Check sheet for the modelled part. Datum: model origin and axes. Units: mm. Round coordinates to 2 decimals unless told otherwise and drop trailing zeros. Write each loop counter-clockwise with the first axis right and the second up, starting at its lowest first coordinate (ties: lowest second). Pieces come first, ordered by that corner, then holes.
Item 1: Cross-section at B-B on y = 104.65. Count the separate pieces of the cut face and the enclosed holes in it, plus the area to 3 significant figures.
Item 2: Go/stop test with flat-tipped pins: pin 1 Ø1.2 at (x, y) = (109, 103) entering from -Z; pin 2 Ø1.2 at (x, y) = (141, 103.5) entering from -Z; pin 3 Ø1 at (y, z) = (104, 218) entering from -X. Record where each tip stops, or that it passes through.
Item 3: Material ranges on line 1 (Z direction, x = 67, y = 103.9); line 2 (Z direction, x = 188.5, y = 103.75); line 3 (Z direction, x = 170.5, y = 101.6), recorded low to high.
Item 4: Cross-section at A-A on x = 77.5. Enter the section's corners in (y, z), plus the area to 3 significant figures.
Item 5: Cross-section at C-C on x = 134. Enter the section's corners in (y, z).
from build123d import *

# Parameters (mm, degrees)
SKETCH1_W           = 10.75
SKETCH1_H           = 4
SKETCH1_R           = 1.6
SKETCH1_R_2         = 9
SKETCH1_R_3         = 8.5
BOSS_EXTRUDE1_DEPTH = 4
FILLET2_R           = 3


with BuildPart() as part:
    # Sketch1 → Boss-Extrude1 (new body)
    with BuildSketch(Plane(origin=(0, 101.33365526, 0), x_dir=(1, 0, 0), z_dir=(0, 1, 0))):
        with BuildLine():
            Line((99.937186027, -237.061198021), (99.937186027, -207.061198021))
            Line((99.937186027, -207.061198021), (112.937186027, -207.061198021))
            Line((112.937186027, -207.061198021), (112.937186027, -193.701198021))
            Line((112.937186027, -193.701198021), (116.937186027, -193.701198021))
            Line((116.937186027, -193.701198021), (116.937186027, -193.724971735))
            ThreePointArc((116.937186027, -193.724971735), (120.422613168, -188.743411519), (125.937186027, -186.183405518))
            Line((125.937186027, -186.183405518), (125.937186027, -182.011198021))
            Line((125.937186027, -182.011198021), (129.937186027, -182.011198021))
            Line((129.937186027, -182.011198021), (129.937186027, -186.183405518))
            ThreePointArc((129.937186027, -186.183405518), (135.451758886, -188.743411519), (138.937186027, -193.724971735))
            Line((138.937186027, -193.724971735), (138.937186027, -193.701198021))
            Line((138.937186027, -193.701198021), (142.937186027, -193.701198021))
            Line((142.937186027, -193.701198021), (142.937186027, -207.061198021))
            Line((142.937186027, -207.061198021), (155.937186027, -207.061198021))
            Line((155.937186027, -207.061198021), (155.937186027, -237.061198021))
            Line((155.937186027, -237.061198021), (180.437186027, -237.061198021))
            ThreePointArc((180.437186027, -237.061198021), (216.632797463, -160.061198021), (180.437186027, -83.061198021))
            Line((180.437186027, -83.061198021), (155.937186027, -83.061198021))
            Line((155.937186027, -83.061198021), (155.937186027, -113.061198021))
            Line((155.937186027, -113.061198021), (142.937186027, -113.061198021))
            Line((142.937186027, -113.061198021), (142.937186027, -126.421198021))
            Line((142.937186027, -126.421198021), (138.937186027, -126.421198021))
            Line((138.937186027, -126.421198021), (138.937186027, -126.397424307))
            ThreePointArc((138.937186027, -126.397424307), (135.451758886, -131.378984523), (129.937186027, -133.938990524))
            Line((129.937186027, -133.938990524), (129.937186027, -138.111198021))
            Line((129.937186027, -138.111198021), (125.937186027, -138.111198021))
            Line((125.937186027, -138.111198021), (125.937186027, -133.938990524))
            ThreePointArc((125.937186027, -133.938990524), (120.422613168, -131.378984523), (116.937186027, -126.397424307))
            Line((116.937186027, -126.397424307), (116.937186027, -126.421198021))
            Line((116.937186027, -126.421198021), (112.937186027, -126.421198021))
            Line((112.937186027, -126.421198021), (112.937186027, -113.061198021))
            Line((112.937186027, -113.061198021), (99.937186027, -113.061198021))
            Line((99.937186027, -113.061198021), (99.937186027, -83.061198021))
            Line((99.937186027, -83.061198021), (52.828408899, -83.061198021))
            ThreePointArc((52.828408899, -83.061198021), (16.632797463, -160.061198021), (52.828408899, -237.061198021))
            Line((52.828408899, -237.061198021), (99.937186027, -237.061198021))
        make_face()
        with Locations((175.062186027, -95.061198021)):
            Rectangle(SKETCH1_W, SKETCH1_H, mode=Mode.SUBTRACT)
        Polygon((56.893376849, -220.531213103), (49.699978846, -227.477796808), (46.921345364, -224.600437606), (54.114743367, -217.653853902), align=None, mode=Mode.SUBTRACT)
        with Locations((104.217909851, -196.061198021)):
            Circle(SKETCH1_R, mode=Mode.SUBTRACT)
        Polygon((116.937186027, -142.561198021), (116.937186027, -177.561198021), (112.937186027, -177.561198021), (112.937186027, -162.061198021), (106.437186027, -162.061198021), (106.437186027, -158.061198021), (112.937186027, -158.061198021), (112.937186027, -142.561198021), align=None, mode=Mode.SUBTRACT)
        with Locations((175.062186027, -225.061198021)):
            Rectangle(SKETCH1_W, SKETCH1_H, mode=Mode.SUBTRACT)
        with Locations((175.937186027, -203.061198021)):
            Circle(SKETCH1_R_2, mode=Mode.SUBTRACT)
        Polygon((192.781361608, -217.850313996), (189.504753431, -215.55600825), (191.799059176, -212.279400073), (195.075667353, -214.573705818), align=None, mode=Mode.SUBTRACT)
        Polygon((201.615472458, -203.246431106), (197.990241309, -201.555958059), (199.680714356, -197.930726911), (203.305945504, -199.621199958), align=None, mode=Mode.SUBTRACT)
        with Locations((162.937186027, -190.561198021)):
            Circle(SKETCH1_R, mode=Mode.SUBTRACT)
        Polygon((138.937186027, -142.561198021), (142.937186027, -142.561198021), (142.937186027, -158.061198021), (149.437186027, -158.061198021), (149.437186027, -162.061198021), (142.937186027, -162.061198021), (142.937186027, -177.561198021), (138.937186027, -177.561198021), align=None, mode=Mode.SUBTRACT)
        with Locations((188.937186027, -190.561198021)):
            Circle(SKETCH1_R, mode=Mode.SUBTRACT)
        Polygon((173.937186027, -138.161198021), (173.937186027, -134.961198021), (177.937186027, -134.961198021), (177.937186027, -138.161198021), (187.387186027, -138.161198021), (187.387186027, -158.061198021), (188.887186027, -158.061198021), (188.887186027, -162.061198021), (187.387186027, -162.061198021), (187.387186027, -181.961198021), (177.937186027, -181.961198021), (177.937186027, -185.161198021), (173.937186027, -185.161198021), (173.937186027, -181.961198021), (164.487186027, -181.961198021), (164.487186027, -138.161198021), align=None, mode=Mode.SUBTRACT)
        Polygon((211.08596232, -170.585781918), (207.101183528, -170.237158947), (207.449806499, -166.252380154), (211.434585291, -166.601003125), align=None, mode=Mode.SUBTRACT)
        with BuildLine():
            ThreePointArc((30.129612814, -122.561198021), (32.472758565, -116.904343772), (38.129612814, -114.561198021))
            Line((38.129612814, -114.561198021), (46.129612814, -114.561198021))
            ThreePointArc((46.129612814, -114.561198021), (51.786467064, -116.904343772), (54.129612814, -122.561198021))
            Line((54.129612814, -122.561198021), (54.129612814, -197.561198021))
            ThreePointArc((54.129612814, -197.561198021), (51.786467064, -203.21805227), (46.129612814, -205.561198021))
            Line((46.129612814, -205.561198021), (38.129612814, -205.561198021))
            ThreePointArc((38.129612814, -205.561198021), (32.472758565, -203.21805227), (30.129612814, -197.561198021))
            Line((30.129612814, -197.561198021), (30.129612814, -122.561198021))
        make_face(mode=Mode.SUBTRACT)
        with BuildLine():
            Line((58.629612814, -206.061198021), (58.629612814, -114.061198021))
            Line((58.629612814, -114.061198021), (80.629612814, -114.061198021))
            ThreePointArc((80.629612814, -114.061198021), (82.750933158, -114.939877677), (83.629612814, -117.061198021))
            Line((83.629612814, -117.061198021), (83.629612814, -203.061198021))
            ThreePointArc((83.629612814, -203.061198021), (82.750933158, -205.182518365), (80.629612814, -206.061198021))
            Line((80.629612814, -206.061198021), (58.629612814, -206.061198021))
        make_face(mode=Mode.SUBTRACT)
        with Locations((104.217909851, -124.061198021)):
            Circle(SKETCH1_R, mode=Mode.SUBTRACT)
        Polygon((54.114743367, -102.46854214), (46.921345364, -95.521958436), (49.699978846, -92.644599234), (56.893376849, -99.591182939), align=None, mode=Mode.SUBTRACT)
        with Locations((127.937186027, -160.061198021)):
            Circle(SKETCH1_R_3, mode=Mode.SUBTRACT)
        with Locations((162.937186027, -129.561198021)):
            Circle(SKETCH1_R, mode=Mode.SUBTRACT)
        Polygon((211.434585291, -153.521392917), (207.449806499, -153.870015888), (207.101183528, -149.885237095), (211.08596232, -149.536614124), align=None, mode=Mode.SUBTRACT)
        with Locations((188.937186027, -129.561198021)):
            Circle(SKETCH1_R, mode=Mode.SUBTRACT)
        with Locations((175.937186027, -117.061198021)):
            Circle(SKETCH1_R_2, mode=Mode.SUBTRACT)
        Polygon((203.305945504, -120.501196084), (199.680714356, -122.191669131), (197.990241309, -118.566437983), (201.615472457, -116.875964936), align=None, mode=Mode.SUBTRACT)
        Polygon((195.075667353, -105.548690224), (191.799059176, -107.842995969), (189.504753431, -104.566387792), (192.781361608, -102.272082046), align=None, mode=Mode.SUBTRACT)
    extrude(amount=BOSS_EXTRUDE1_DEPTH)

    # Fillet2
    fillet2_edges = [part.edges().sort_by_distance(p)[0] for p in [
        (99.937186027, 103.33365526, 83.061198021),
        (99.937186027, 103.33365526, 113.061198021),
        (155.937186027, 103.33365526, 113.061198021),
        (155.937186027, 103.33365526, 83.061198021),
        (155.937186027, 103.33365526, 237.061198021),
        (155.937186027, 103.33365526, 207.061198021),
        (99.937186027, 103.33365526, 207.061198021),
        (99.937186027, 103.33365526, 237.061198021),
    ]]
    fillet(fillet2_edges, radius=FILLET2_R)


solid = part.part
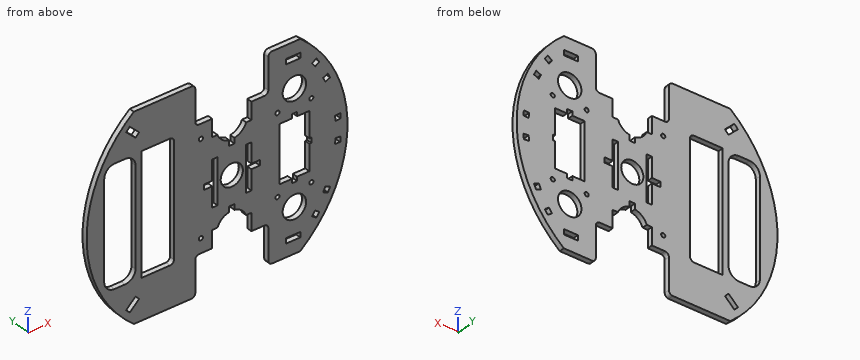
Response values:
1. separate pieces: 1
1. enclosed holes: 24
1. area: 16,100 mm2
2. pin 1: stops at z = 113.06
2. pin 2: stops at z = 126.42
2. pin 3: stops at x = 34.77
3. line 1: z = 83.06 to 114.06, 206.06 to 237.06
3. line 2: z = 90.53 to 128.02, 131.1 to 158.06, 162.06 to 189.02, 192.1 to 229.6
3. line 3: z = 83.06 to 93.06, 97.06 to 109.89, 124.23 to 138.16, 181.96 to 195.89, 210.23 to 223.06, 227.06 to 237.06
4. outline: (101.33, 83.06) - (105.33, 83.06) - (105.33, 114.06) - (101.33, 114.06) - close; (101.33, 206.06) - (105.33, 206.06) - (105.33, 237.06) - (101.33, 237.06) - close
4. area: 248 mm2
5. outline: (101.33, 132.42) - (105.33, 132.42) - (105.33, 154.1) - (101.33, 154.1) - close; (101.33, 166.02) - (105.33, 166.02) - (105.33, 187.7) - (101.33, 187.7) - close
